```python
from build123d import *

# Parameters (mm, degrees)
RESSALTO_EXTRUS_O1_DEPTH          = 3.5
RESSALTO_EXTRUS_O2_DEPTH          = 1.8
ESBO_O5_W                         = 49.5
ESBO_O5_H                         = 3
RESSALTO_EXTRUS_O3_DEPTH          = 12
ESBO_O6_W                         = 1.5
ESBO_O6_H                         = 17.8
RESSALTO_EXTRUS_O4_DEPTH          = 1.8
ESBO_O7_R                         = 1
CORTE_EXTRUS_O2_DEPTH             = 45.583701426
CORTE_EXTRUS_O4_DEPTH             = 45.583701426
RESSALTO_EXTRUS_O5_DEPTH          = 8
RESSALTO_EXTRUS_O6_DEPTH          = 8
ESBO_O12_W                        = 11.60028147
ESBO_O12_H                        = 18
ESBO_O12_W_2                      = 11.59971853
RESSALTO_EXTRUS_O7_DEPTH          = 2
ESBO_O4_R                         = 1
CORTE_EXTRUS_O1_DEPTH             = 10
ESBO_O14_W                        = 23.3
ESBO_O14_H                        = 21.5
RESSALTO_EXTRUS_O8_DEPTH          = 5
CORTE_EXTRUS_O5_REACH             = 50.124
CORTE_EXTRUS_O5_DIRECTION_2_DEPTH = 10
CORTE_EXTRUS_O6_REACH             = 42.044
ESBO_O16_R                        = 1.35
FILETE1_R                         = 5


with BuildPart() as part:
    # Esbo_o1 → Ressalto-extrus_o1 (new body)
    with BuildSketch(Plane.XY):
        Polygon((-13.15, -9.5), (13.15, -9.5), (13.15, 6.5), (13.15, 26.3), (-13.15, 26.3), (-13.15, 6.5), align=None)
    extrude(amount=RESSALTO_EXTRUS_O1_DEPTH)

    # Esbo_o2 → Ressalto-extrus_o2 (add)
    with BuildSketch(Plane.XY.offset(3.5)):
        Polygon((24.75028147, 8.5), (11.65, 8.5), (11.65, 4.8), (-11.65, 4.8), (-11.65, 8.5), (-24.74971853, 8.5), (-24.74971853, -9.5), (-11.65, -9.5), (10.65, -9.5), (24.75028147, -9.5), align=None)
    extrude(amount=RESSALTO_EXTRUS_O2_DEPTH)

    # Esbo_o5 → Ressalto-extrus_o3 (add)
    with BuildSketch(Plane.XY.offset(5.3)):
        with Locations((0.00028147, -8)):
            Rectangle(ESBO_O5_W, ESBO_O5_H)
    extrude(amount=RESSALTO_EXTRUS_O3_DEPTH)

    # Esbo_o6 → Ressalto-extrus_o4 (add)
    with BuildSketch(Plane.XY.offset(3.5)):
        with Locations((-12.4, 17.4)):
            Rectangle(ESBO_O6_W, ESBO_O6_H)
        with Locations((12.4, 17.4)):
            Rectangle(ESBO_O6_W, ESBO_O6_H)
    extrude(amount=RESSALTO_EXTRUS_O4_DEPTH)

    # Esbo_o7 → Corte-extrus_o2 (cut, through all)
    with BuildSketch(Plane(origin=(0, -6.5, 0), x_dir=(1, 0, 0), z_dir=(0, 1, 0))):
        with Locations(Location((19.237396406, -13.252377825, 0), (0, 0, 270))):
            Circle(ESBO_O7_R)
        with Locations(Location((-19.236833466, -13.252377825, 0), (0, 0, 270))):
            Circle(ESBO_O7_R)
    extrude(amount=-CORTE_EXTRUS_O2_DEPTH, mode=Mode.SUBTRACT)

    # Esbo_o9 → Corte-extrus_o4 (cut, through all)
    with BuildSketch(Plane(origin=(0, -6.5, 0), x_dir=(1, 0, 0), z_dir=(0, 1, 0))):
        Polygon((-5.087829915, -5.323896898), (5.912170085, -5.3), (5.912170085, -14.390715249), (5.912170085, -17.3), (-5.087829915, -17.3), (-5.087829915, -14.390715249), align=None)
    extrude(amount=-CORTE_EXTRUS_O4_DEPTH, mode=Mode.SUBTRACT)

    # Esbo_o10 → Ressalto-extrus_o5 (add)
    with BuildSketch(Plane(origin=(24.75028147, 0, 0), x_dir=(0, 0, -1), z_dir=(1, 0, 0))):
        Polygon((-6.3, -6.5), (-5.3, -6.5), (-5.3, -5.5), align=None)
    extrude(amount=-RESSALTO_EXTRUS_O5_DEPTH)

    # Esbo_o11 → Ressalto-extrus_o6 (add)
    with BuildSketch(Plane.ZY.offset(24.74971853)):
        Polygon((5.3, -5.5), (6.3, -6.5), (5.3, -6.5), align=None)
    extrude(amount=-RESSALTO_EXTRUS_O6_DEPTH)

    # Esbo_o12 → Ressalto-extrus_o7 (add)
    with BuildSketch(Plane(origin=(0, 0, 3.5), x_dir=(-1, 0, 0), z_dir=(0, 0, -1))):
        with Locations((-18.950140735, -0.5)):
            Rectangle(ESBO_O12_W, ESBO_O12_H)
        with Locations((18.949859265, -0.5)):
            Rectangle(ESBO_O12_W_2, ESBO_O12_H)
    extrude(amount=RESSALTO_EXTRUS_O7_DEPTH)

    # Esbo_o4 → Corte-extrus_o1 (cut)
    with BuildSketch(Plane.XY.offset(5.3)):
        with Locations((-18.129829915, 0.0659)):
            Circle(ESBO_O4_R)
        with Locations((18.954170085, 0.0659)):
            Circle(ESBO_O4_R)
    extrude(amount=-CORTE_EXTRUS_O1_DEPTH, mode=Mode.SUBTRACT)

    # Esbo_o14 → Ressalto-extrus_o8 (add)
    with BuildSketch(Plane.XY.offset(3.5)):
        with Locations((0, 15.55)):
            Rectangle(ESBO_O14_W, ESBO_O14_H)
    extrude(amount=RESSALTO_EXTRUS_O8_DEPTH)

    # Esbo_o15 → Corte-extrus_o5 (cut, up to next)
    with BuildSketch(Plane(origin=(11.65, 0, 0), x_dir=(0, 0, -1), z_dir=(1, 0, 0)), mode=Mode.PRIVATE) as corte_extrus_o5_sk1:
        Polygon((-8.5, 26.3), (-8.5, 4.8), (-3.930033924, 26.3), align=None)
    corte_extrus_o5_tool1 = extrude(corte_extrus_o5_sk1.sketch, amount=-CORTE_EXTRUS_O5_REACH, mode=Mode.PRIVATE) & part.part
    add(corte_extrus_o5_tool1.solids().sort_by_distance((11.65, 19.133333, 6.976678))[0], mode=Mode.SUBTRACT)

    # Esbo_o15 → Corte-extrus_o5 direction 2 (cut)
    with BuildSketch(Plane(origin=(11.65, 0, 0), x_dir=(0, 0, -1), z_dir=(1, 0, 0))):
        Polygon((-8.5, 26.3), (-8.5, 4.8), (-3.930033924, 26.3), align=None)
    extrude(amount=CORTE_EXTRUS_O5_DIRECTION_2_DEPTH, mode=Mode.SUBTRACT)

    # Corte-extrus_o6: up to this plane
    corte_extrus_o6_end = Plane(origin=(21.65, 4.8, 8.5), z_dir=(0, 0.20791169081775246, 0.9781476007338071))
    # Esbo_o16 → Corte-extrus_o6 (cut, up to the surface)
    with BuildSketch(Plane(origin=(0, 0, 0), x_dir=(-1, 0, 0), z_dir=(0, 0, -1)), mode=Mode.PRIVATE) as corte_extrus_o6_sk1:
        with Locations((7.908, 22.199)):
            Circle(ESBO_O16_R)
    corte_extrus_o6_tool1 = split(extrude(corte_extrus_o6_sk1.sketch, amount=-CORTE_EXTRUS_O6_REACH, mode=Mode.PRIVATE), bisect_by=corte_extrus_o6_end, keep=Keep.BOTH, mode=Mode.PRIVATE)
    add(corte_extrus_o6_tool1.solids().sort_by_distance((-7.908, 22.199, 0))[0], mode=Mode.SUBTRACT)
    # Esbo_o16 → Corte-extrus_o6 (cut, up to the surface)
    with BuildSketch(Plane(origin=(0, 0, 0), x_dir=(-1, 0, 0), z_dir=(0, 0, -1)), mode=Mode.PRIVATE) as corte_extrus_o6_sk2:
        with Locations((-9.11, 9.245)):
            Circle(ESBO_O16_R)
    corte_extrus_o6_tool2 = split(extrude(corte_extrus_o6_sk2.sketch, amount=-CORTE_EXTRUS_O6_REACH, mode=Mode.PRIVATE), bisect_by=corte_extrus_o6_end, keep=Keep.BOTH, mode=Mode.PRIVATE)
    add(corte_extrus_o6_tool2.solids().sort_by_distance((9.11, 9.245, 0))[0], mode=Mode.SUBTRACT)
    # Esbo_o16 → Corte-extrus_o6 (cut, up to the surface)
    with BuildSketch(Plane(origin=(0, 0, 0), x_dir=(-1, 0, 0), z_dir=(0, 0, -1)), mode=Mode.PRIVATE) as corte_extrus_o6_sk3:
        with Locations(Location((9.11, 9.245, 0), (0, 0, 90))):
            Circle(ESBO_O16_R)
    corte_extrus_o6_tool3 = split(extrude(corte_extrus_o6_sk3.sketch, amount=-CORTE_EXTRUS_O6_REACH, mode=Mode.PRIVATE), bisect_by=corte_extrus_o6_end, keep=Keep.BOTH, mode=Mode.PRIVATE)
    add(corte_extrus_o6_tool3.solids().sort_by_distance((-9.11, 9.245, 0))[0], mode=Mode.SUBTRACT)
    # Esbo_o16 → Corte-extrus_o6 (cut, up to the surface)
    with BuildSketch(Plane(origin=(0, 0, 0), x_dir=(-1, 0, 0), z_dir=(0, 0, -1)), mode=Mode.PRIVATE) as corte_extrus_o6_sk4:
        with Locations(Location((-7.908, 22.199, 0), (0, 0, 90))):
            Circle(ESBO_O16_R)
    corte_extrus_o6_tool4 = split(extrude(corte_extrus_o6_sk4.sketch, amount=-CORTE_EXTRUS_O6_REACH, mode=Mode.PRIVATE), bisect_by=corte_extrus_o6_end, keep=Keep.BOTH, mode=Mode.PRIVATE)
    add(corte_extrus_o6_tool4.solids().sort_by_distance((7.908, 22.199, 0))[0], mode=Mode.SUBTRACT)
    # Esbo_o16 → Corte-extrus_o6 (cut, up to the surface)
    with BuildSketch(Plane(origin=(0, 0, 0), x_dir=(-1, 0, 0), z_dir=(0, 0, -1)), mode=Mode.PRIVATE) as corte_extrus_o6_sk5:
        with Locations((-8.509, 15.722)):
            Circle(ESBO_O16_R)
    corte_extrus_o6_tool5 = split(extrude(corte_extrus_o6_sk5.sketch, amount=-CORTE_EXTRUS_O6_REACH, mode=Mode.PRIVATE), bisect_by=corte_extrus_o6_end, keep=Keep.BOTH, mode=Mode.PRIVATE)
    add(corte_extrus_o6_tool5.solids().sort_by_distance((8.509, 15.722, 0))[0], mode=Mode.SUBTRACT)
    # Esbo_o16 → Corte-extrus_o6 (cut, up to the surface)
    with BuildSketch(Plane(origin=(0, 0, 0), x_dir=(-1, 0, 0), z_dir=(0, 0, -1)), mode=Mode.PRIVATE) as corte_extrus_o6_sk6:
        with Locations(Location((8.509, 15.722, 0), (0, 0, 90))):
            Circle(ESBO_O16_R)
    corte_extrus_o6_tool6 = split(extrude(corte_extrus_o6_sk6.sketch, amount=-CORTE_EXTRUS_O6_REACH, mode=Mode.PRIVATE), bisect_by=corte_extrus_o6_end, keep=Keep.BOTH, mode=Mode.PRIVATE)
    add(corte_extrus_o6_tool6.solids().sort_by_distance((-8.509, 15.722, 0))[0], mode=Mode.SUBTRACT)

    # Filete1
    filete1_edges = [part.edges().sort_by_distance(p)[0] for p in [
        (24.75028147, 8.5, 3.4),
        (-24.74971853, 8.5, 3.4),
        (-13.15, 26.3, 1.965016962),
        (13.15, 26.3, 1.965016962),
    ]]
    fillet(filete1_edges, radius=FILETE1_R)


solid = part.part
```
CAD build for the part. Positions are in the model's coordinates, mm. A direction names the side the tool comes from. Coordinates: 2 decimals unless noted, no trailing zeros. Order: outer loops, then holes, each group sorted by start corner. A loop starts at its lowest first (then second) coordinate and runs counter-clockwise, first axis right, second up. Notation, with made-up numbers: (30.5, 76.5) - (60.5, 76.5) arc R29 cw to (60.5, 107.5) - close; hole circle Ø3 at (-9.5, -4.5). An arc over 180 degrees is marked (long way). Use a Markdown table: item, result. Add a question column.
(1) Which spindle directions (+Z, -Z, +X, -X, +Y, -Y) get a long thin tool onto all of the face, cutting with end or side? Do faces 5 (the face through (11.65, 11, 7)), 6 (the face through (16.75, -6.2, 5.6)), 7 (the face through (-20, 0, 1.5)), 8 (the face through (17.7, -0.4, 1.5)). Say none if no direction does.
(2) Saw through at C-C (y = -4). Give the cut face in (x, z).
(3) Flat gauge pins, fed straight in: pin 1 (2 mm diameter, centred on x = -18, y = -4.5, fed in from -Z); pin 2 (9.5 mm diameter, centred on x = 19, z = 9.5, fed in from +Y); pin 3 (13 mm diameter, centred on x = -11, y = 8.5, fed in from +Z); pin 4 (3 mm diameter, centred on x = 19.24, z = 13.25, fed in from -Y). Where does each tip first touch, or does it go through?
(4) Saw through at D-D (z = 2.25). Count the separate pieces of the cut face and the enclosed holes in it, then the cut area to 3 significant figures.
(5) Drill centre lines: line 1 along Y through (x, z) = (-17, 2); line 2 along X through (y, z) = (13, 1.25); line 3 along Y through (x, z) = (21.5, 11.25). Where is each one in solid material? Low to high. Write a range as [from, to].
(6) Pull direction Y, two halves, no side cores. Call faces 1 (the face through (-5.088, -8, 11)), 2 (the face through (-23.32, 7, 3.37)), 3 (the face through (-19.13, 0.11, 3.43)), 4 (the face through (7.97, 20.85, 2.52)): +Y half, -Y half, draft (parallel to the pull), parting line (faces both ways), or undercut.
(7) Saw through at B-B (x = -14.5). Give the cut face in (y, z), then the cut area to 3 significant figures.
(8) Saw through at A-A (z = 10.75). Give the cut face in (x, y).
Solved:
| question | item | result |
|---|---|---|
| 1 | face 5 | +Z, +X, +Y |
| 1 | face 6 | +Z, +Y |
| 1 | face 7 | -Z, -X, +Y, -Y |
| 1 | face 8 | -Z, +X, +Y, -Y |
| 2 | outline | (-24.75, 1.5) - (-13.15, 1.5) - (-13.15, 0) - (13.15, 0) - (13.15, 1.5) - (24.75, 1.5) - (24.75, 5.3) - (-24.75, 5.3) - close |
| 3 | pin 1 | stops at z = 1.5 |
| 3 | pin 2 | stops at y = 8.5 |
| 3 | pin 3 | stops at z = 8.5 |
| 3 | pin 4 | stops at y = -9.5 |
| 4 | separate pieces | 1 |
| 4 | enclosed holes | 8 |
| 4 | area | 1,300 mm² |
| 5 | line 1 | y = [-9.5, 8.5] |
| 5 | line 2 | x = [-13.15, 13.15] |
| 5 | line 3 | y = [-9.5, -6.5] |
| 6 | face 1 | draft |
| 6 | face 2 | +Y half |
| 6 | face 3 | undercut |
| 6 | face 4 | undercut |
| 7 | outline | (-9.5, 1.5) - (8.5, 1.5) - (8.5, 5.3) - (-6.5, 5.3) - (-6.5, 17.3) - (-9.5, 17.3) - close |
| 7 | area | 104 mm² |
| 8 | outline | (-24.75, -9.5) - (-5.09, -9.5) - (-5.09, -6.5) - (-24.75, -6.5) - close; (5.91, -9.5) - (24.75, -9.5) - (24.75, -6.5) - (5.91, -6.5) - close |
